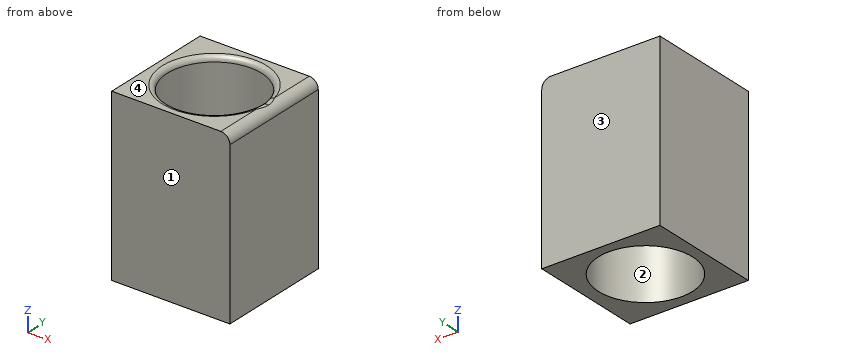
```python
from build123d import *

# Parameters (mm, degrees)
F0_W     = 127.844266
F0_H     = 124.537945
F0_R     = 50.933349
F1_DEPTH = 185.166
F2_R     = 9.811364
F3_R     = 5.518892


with BuildPart() as f1:
    # F0 (on Top) → F1 (new body)
    with BuildSketch(Plane.XY):
        with Locations((0.874225, -0.474699)):
            Rectangle(F0_W, F0_H)
        Circle(F0_R, mode=Mode.SUBTRACT)
    extrude(amount=F1_DEPTH)

    # F2
    f2_edges = [f1.edges().sort_by_distance(p)[0] for p in [
        (64.796358, -0.474699, 185.166),
    ]]
    fillet(f2_edges, radius=F2_R)

    # F3
    f3_edges = [f1.edges().sort_by_distance(p)[0] for p in [
        (-50.933349, 0, 185.166),
    ]]
    fillet(f3_edges, radius=F3_R)


solid = f1.part
```
Read the model definition and answer for the solid it produces. Units are mm, in the model's axes. Face numbers are marked on the shaded views. Round coordinates to 2 decimals unless told otherwise and drop trailing zeros. Write each loop counter-clockwise with the first axis right and the second up, starting at its lowest first coordinate (ties: lowest second). Pieces come first, ordered by that corner, then holes. Notation, with made-up numbers: M 62,-30.5 L 121,-30.5 A16 ccw 121,-7.5 Z; hole C 68.25,70.5 d7. An arc over 180 degrees is marked long. One line per item, written item: value.
Q1. Find section B-B on z = 64.5. Write down the section's boundary in (x, y), plus the area to 3 significant figures.
Data:
outline: M -63.05,-62.74 L 64.8,-62.74 L 64.8,61.79 L -63.05,61.79 Z; hole C 0,0 d101.87
area: 7,770 mm2
Q2. Find section A-A on x = 0. Write down the section's boundary in (y, z).
Data:
outline: M -62.74,0 L -50.93,0 L -50.93,179.65 A5.52 ccw -56.45,185.17 L -62.74,185.17 Z; M 50.93,0 L 61.79,0 L 61.79,185.17 L 56.45,185.17 A5.52 ccw 50.93,179.65 Z
Q3. For a pull along Y with two mould halves and no side action, classify the marked faces 1, 2, 3 and 4 as +Y half, -Y half, draft (parallel to the pull), parting line (faces both ways), or undercut.
Data:
face 1: -Y half
face 2: undercut
face 3: +Y half
face 4: draft
Q4. Straight lines are drawn through the part: line 1 (Y direction, x = 1, z = 56.5); line 2 (X direction, y = -0.5, z = 63); line 3 (Y direction, x = 25, z = 136). For each, find the intervals that lie inside material, in ascending order. Write a range as [from, to].
Data:
line 1: [-62.74, -50.92], [50.92, 61.79]
line 2: [-63.05, -50.93], [50.93, 64.8]
line 3: [-62.74, -44.38], [44.38, 61.79]
